from build123d import *

# Parameters (mm, degrees)
F0_W     = 76.2
F0_H     = 50.8
F1_DEPTH = 25.4
F2_DEPTH = 25.4
F3_R     = 25.39999
F4_T     = -2.54
F6_D     = 3.81
F8_DEPTH = 25.4


# Not quite as in the source:
# - a fillet or chamfer is up to 0.001 mm smaller than in the source, because OpenCascade refuses the exact size


with BuildPart() as f1:
    # F0 (on Top) → F1 (new body)
    with BuildSketch(Plane.XY):
        Rectangle(F0_W, F0_H)
    extrude(amount=F1_DEPTH)

    # F2 (add): a face of the model
    f2_faces = [f1.faces().sort_by_distance(p)[0] for p in [
        (0, 0, 0),
    ]]
    extrude(f2_faces, amount=F2_DEPTH)

    # F3 (radius 25.4 in the source; OpenCascade refuses exactly that, so slightly less here)
    f3_edges = [f1.edges().sort_by_distance(p)[0] for p in [
        (0, -25.4, -25.4),
        (38.1, 0, -25.4),
        (0, 25.4, -25.4),
        (-38.1, 0, -25.4),
    ]]
    fillet(f3_edges, radius=F3_R)

    # F4
    f4_openings = [f1.faces().sort_by_distance(p)[0] for p in [
        (0, 0, 25.4),
    ]]
    offset(amount=F4_T, openings=f4_openings)

    # F6 (through all)
    with Locations(Plane.XY):
        with Locations((0, 0)):
            Hole(F6_D / 2)

    # F7 (on face) → F8 (cut)
    with BuildSketch(Plane.XY.offset(25.4)):
        Polygon((-35.56, -22.86), (-38.1, -25.4), (38.1, -25.4), (35.56, -22.86), align=None)
    extrude(amount=-F8_DEPTH, mode=Mode.SUBTRACT)


solid = f1.part
Can you work these out from the model? Positions are in its coordinate system, mm. A direction names the side the tool comes from. Round coordinates to 2 decimals unless told otherwise and drop trailing zeros. Order: outer loops, then holes, each group sorted by start corner. A loop starts at its lowest first (then second) coordinate and runs counter-clockwise, first axis right, second up. Notation, with made-up numbers: (-5, -11.5) -> (3, -11.5) arc R18 ccw to (3, 21.5) -> close; hole circle Ø3 at (-10.75, 78). An arc over 180 degrees is marked (long way). Write each question's results on one line, items separated by ' | '. Start each with the question number.
Item 1: Thinking about a two-plate mould opening in Y: for faces 4 (the cylindrical face through (-31.569, 0.32, -12.905)), 5 (the flat face through (38.1, 0, 13)), 6 (the cylindrical face through (0.533, 20.965, -14.339)), which applies, +Y half, -Y half, draft (parallel to the pull), parting line (faces both ways), or undercut?
Item 2: If we section it at D-D, the plane y = -17: Write out the boundary of the cut face in (x, z), then the cut area to 3 significant figures.
Item 3: If we section it at C-C, the plane z = 21: Write out the boundary of the cut face in (x, y), then the cut area to 3 significant figures.
Item 4: If we section it at B-B, the plane z = -8: Write out the boundary of the cut face in (x, y), then the cut area to 3 significant figures.
Item 5: Which directions (+Z, -Z, +X, -X, +Y, -Y) give clear straight access to the entire face, cutting with the end or side of a thin tool? Please do faces 1 (the flat face through (-1, -24, 0)), 2 (the cylindrical face through (-33.665, 0.356, -14.339)), 3 (the cylindrical face through (31.569, 0.32, -12.905)).
Item 6: Please list where these lines run through material, in increasing order: L1, parallel to X at y = -5, z = 6; L2, parallel to Y at x = 17, z = 0.5; L3, parallel to Y at x = 15.5, z = -10.
Item 7: Will these pins go through, and if not, where does the flat tip stop? pin 1 (5 mm diameter, centred on x = 9, y = 14.5, fed in from -Z); pin 2 (6 mm diameter, centred on x = 0, y = 0, fed in from +Z); pin 3 (6 mm diameter, centred on x = -13.5, y = -20, fed in from -Z); pin 4 (8 mm diameter, centred on x = -1, z = 2.5, fed in from -Y).
Results:
1) face 4: undercut | face 5: draft | face 6: +Y half
2) outline: (-38.1, 0) arc R25.4 ccw to (-29.7, -18.87) -> (29.7, -18.87) arc R25.4 ccw to (38.1, 0) -> (38.1, 25.4) -> (35.56, 25.4) -> (35.56, 0) arc R22.86 cw to (29.7, -15.28) -> (-29.7, -15.28) arc R22.86 cw to (-35.56, 0) -> (-35.56, 25.4) -> (-38.1, 25.4) -> close | area: 439 mm2
3) outline: (-38.1, -25.4) -> (-35.56, -22.86) -> (-35.56, 22.86) -> (35.56, 22.86) -> (35.56, -22.86) -> (38.1, -25.4) -> (38.1, 25.4) -> (-38.1, 25.4) -> close | area: 432 mm2
4) outline: (-36.81, -24.11) -> (36.81, -24.11) -> (36.81, 24.11) -> (-36.81, 24.11) -> close; hole (-34.11, -21.41) -> (34.11, -21.41) -> (34.11, 21.41) -> (-34.11, 21.41) -> close | area: 627 mm2
5) face 1: +Z, -Y | face 2: -Z, -X, +Y, -Y | face 3: +Z
6) L1: x = -38.1 to -35.56, 35.56 to 38.1 | L2: y = 22.86 to 25.4 | L3: y = -23.35 to -20.56, 20.56 to 23.35
7) pin 1: stops at z = -22.39 | pin 2: stops at z = -22.66 | pin 3: stops at z = -18.87 | pin 4: stops at y = -25.4
